For this review, take the finished solid that the model builds, in its own axes (mm). Coordinates: 2 decimals unless noted, no trailing zeros. Loops run counter-clockwise (first coordinate to the right, second up) from the corner with the lowest first, then second, coordinate; pieces in that order, holes last.
1. Take a section at B-B, the plane y = -8. State the section outline as (x, z) points.
2. Mouldability with a two-part tool opening along Y and no side actions: class faces 1 (the face through (30.376, 24.819, 0.789)), 2 (the face through (-11, -2, 0)) as pulls with the +Y half, pulls with the -Y half, needs draft (parallel to the pull), parting line crosses it, or undercut.
3. Take a section at A-A, the plane x = -17.5. State the section outline as (y, z) points, then the cut area to 3 significant figures.
4. To check wall thickness, follow probe 1 along Y at (x, z) = (-18.5, 0.9); probe 2 along X at (y, z) = (13, 0.3); probe 3 along X at (y, z) = (23, 0.3). State the ranges of each line that lie inside material, in increasing order.
5. Take a section at C-C, the plane z = 0.45. Count the separate pieces of the cut face and the enclosed holes in it, then the cut area to 3 significant figures.
```python
from build123d import *

# Parameters (mm, degrees)
SKETCH_2_W          = 90
SKETCH_2_H          = 60
EXTRUDE_1_DEPTH     = 1.6
SKETCH_3_R          = 1.5
SKETCH_3_W          = 76
SKETCH_3_H          = 20
CUT_EXTRUDE_1_DEPTH = 2.6


with BuildPart() as part:
    # ｽｹｯﾁ2 → ﾎﾞｽ - 押し出し1 (new body)
    with BuildSketch(Plane.XY):
        with Locations((-10.192982456, -2.631578947)):
            Rectangle(SKETCH_2_W, SKETCH_2_H)
    extrude(amount=EXTRUDE_1_DEPTH)

    # ｽｹｯﾁ3 → ｶｯﾄ - 押し出し1 (cut, through all)
    with BuildSketch(Plane(origin=(0, 0, 0), x_dir=(-1, 0, 0), z_dir=(0, 0, -1))):
        with Locations((47.192982456, -2.631578947)):
            Circle(SKETCH_3_R)
        with Locations((-26.807017544, -2.631578947)):
            Circle(SKETCH_3_R)
        with Locations((52.192982456, 24.368421053)):
            Circle(SKETCH_3_R)
        with Locations((-31.807017544, 24.368421053)):
            Circle(SKETCH_3_R)
        with Locations((-31.807017544, -29.631578947)):
            Circle(SKETCH_3_R)
        with Locations((52.192982456, -29.631578947)):
            Circle(SKETCH_3_R)
        with Locations((10.192982456, 10.368421053)):
            Rectangle(SKETCH_3_W, SKETCH_3_H)
        with Locations((10.192982456, -15.631578947)):
            Rectangle(SKETCH_3_W, SKETCH_3_H)
    extrude(amount=-CUT_EXTRUDE_1_DEPTH, mode=Mode.SUBTRACT)


solid = part.part
```
Results list:
1. outline: (-55.19, 0) - (-48.19, 0) - (-48.19, 1.6) - (-55.19, 1.6) - close; (27.81, 0) - (34.81, 0) - (34.81, 1.6) - (27.81, 1.6) - close
2. face 1: undercut
2. face 2: needs draft
3. outline: (-32.63, 0) - (-25.63, 0) - (-25.63, 1.6) - (-32.63, 1.6) - close; (-5.63, 0) - (0.37, 0) - (0.37, 1.6) - (-5.63, 1.6) - close; (20.37, 0) - (27.37, 0) - (27.37, 1.6) - (20.37, 1.6) - close
3. area: 32.0 mm2
4. probe 1: y = -32.63 to -25.63, -5.63 to 0.37, 20.37 to 27.37
4. probe 2: x = -55.19 to -48.19, 27.81 to 34.81
4. probe 3: x = -55.19 to -52.81, -51.58 to 31.19, 32.42 to 34.81
5. separate pieces: 1
5. enclosed holes: 8
5. area: 2,320 mm2
